Geometry check sheet. Reference: the model listing, model coordinates, mm. Face numbers are marked on the shaded views. A direction names the side the tool comes from. Round coordinates to 2 decimals unless told otherwise and drop trailing zeros. Order: outer loops, then holes, each group sorted by start corner. A loop starts at its lowest first (then second) coordinate and runs counter-clockwise, first axis right, second up. Notation, with made-up numbers: (87.25, -20) - (105.25, -20) arc R19 cw to (105.25, -1) - close; hole circle Ø4 at (16.25, -38). An arc over 180 degrees is marked (long way). Return JSON: item names as keys, results as strings. Group by question number.
Q1. Sectioned sample at B-B, the plane y = 24. Record the cut outline in (x, z).
Q2. Draft check along X on the marked faces 5, 6 and 7. Enter one of: pulls with the +X half, pulls with the -X half, needs draft (parallel to the pull), parting line crosses it, or undercut.
Q3. Sectioned sample at A-A, the plane z = 0. Record the cut outline in (x, y), then the cut area to 3 significant figures.
Q4. Gauge pin test, flat ends, axial feed: pin 1 Ø9.5 at (y, z) = (30, 19) entering from +X; pin 2 Ø10 at (x, z) = (39.5, -13.5) entering from +Y. Record the tip position at first contact, or that the pin passes through.
Q5. Sectioned sample at D-D, the plane y = 5. Record the cut outline in (x, z).
Q6. Material ranges on line 1 along Y through (x, z) = (-35, -15); line 2 along Z through (x, y) = (-18, 50); line 3 along Y through (x, z) = (12, -10.5), recorded low to high.
Q7. Sectioned sample at C-C, the plane x = -35. Record the cut outline in (y, z).
Q8. Tool access check on the marked faces 1, 2, 3 and 4. Record the directions out of +Z, -Z, +X, -X, +Y, -Y that give a thin tool (end or side, any length) a straight path to the whole face; none if there is none.
```python
from build123d import *

# Parameters (mm, degrees)
SKETCH3_R           = 22
BOSS_EXTRUDE1_DEPTH = 16
CUT_EXTRUDE1_DEPTH  = 16
BOSS_EXTRUDE2_DEPTH = 12
FILLET1_R           = 2


with BuildPart() as part:
    # Sketch3 → Boss-Extrude1 (new body)
    with BuildSketch(Plane(origin=(0, 0, 0), x_dir=(1, 0, 0), z_dir=(0, 1, 0))):
        with BuildLine():
            Line((-59, -22), (37, -22))
            ThreePointArc((37, -22), (15, 0), (37, 22))
            Line((37, 22), (-59, 22))
            Line((-59, 22), (-59, -22))
        make_face()
        with Locations((37, 0)):
            Circle(SKETCH3_R)
    extrude(amount=BOSS_EXTRUDE1_DEPTH)

    # Sketch4 → Cut-Extrude1 (cut)
    with BuildSketch(Plane(origin=(0, 16, 0), x_dir=(1, 0, 0), z_dir=(0, 1, 0))):
        with BuildLine():
            Line((37, -8), (13, -8))
            ThreePointArc((13, -8), (5, 0), (13, 8))
            Line((13, 8), (37, 8))
            ThreePointArc((37, 8), (45, 0), (37, -8))
        make_face()
    extrude(amount=-CUT_EXTRUDE1_DEPTH, mode=Mode.SUBTRACT)

    # Sketch5 → Boss-Extrude2 (add)
    with BuildSketch(Plane.XY.offset(22)):
        with BuildLine():
            Line((-59, 40), (-59, 16))
            Line((-59, 16), (-11, 16))
            Line((-11, 16), (-11, 40))
            Line((-11, 40), (-11.018613653, 40))
            ThreePointArc((-11.018613653, 40), (-35, 16.018613653), (-58.981386347, 40))
            Line((-58.981386347, 40), (-59, 40))
        make_face()
        with BuildLine():
            ThreePointArc((-11.018613653, 40), (-35, 63.981386347), (-58.981386347, 40))
            Line((-58.981386347, 40), (-45, 40))
            ThreePointArc((-45, 40), (-35, 50), (-25, 40))
            Line((-25, 40), (-11.018613653, 40))
        make_face()
        with BuildLine():
            Line((-45, 40), (-58.981386347, 40))
            ThreePointArc((-58.981386347, 40), (-35, 16.018613653), (-11.018613653, 40))
            Line((-11.018613653, 40), (-25, 40))
            ThreePointArc((-25, 40), (-35, 30), (-45, 40))
        make_face()
    boss_extrude2 = extrude(amount=-BOSS_EXTRUDE2_DEPTH)

    # Mirror1: Boss-Extrude2 across plane
    add(boss_extrude2.mirror(Plane.XY))

    # Fillet1
    fillet1_edges = [part.edges().sort_by_distance(p)[0] for p in [
        (-11, 16, 16),
        (-35, 16, 10),
        (-35, 16, -10),
        (-11, 16, -16),
    ]]
    fillet(fillet1_edges, radius=FILLET1_R)


solid = part.part
```
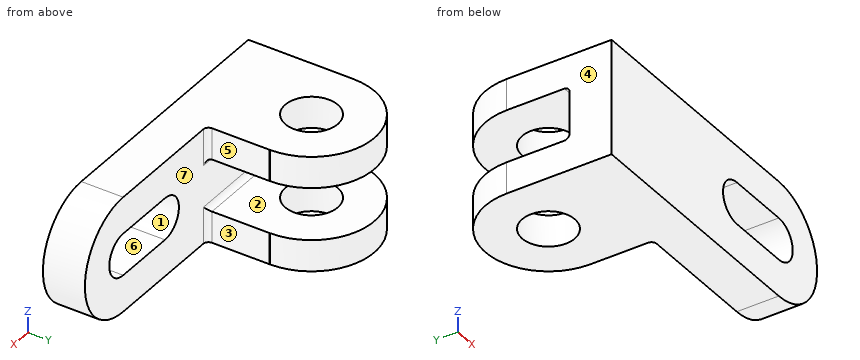
Reply:
{
 "1": {"outline": "(-59, -22) - (-11, -22) - (-11, -10) - (-59, -10) - close; (-59, 10) - (-11, 10) - (-11, 22) - (-59, 22) - close"},
 "2": {"face 5": "pulls with the +X half", "face 6": "undercut", "face 7": "needs draft"},
 "3": {"outline": "(-59, 0) - (5, 0) - (5, 16) - (-59, 16) - close; (45, 0) - (59, 0) - (59, 16) - (45, 16) - close", "area": "1,250 mm^2"},
 "4": {"pin 1": "x = -11", "pin 2": "y = 16"},
 "5": {"outline": "(-59, -22) - (37, -22) arc R22 ccw to (37, 22) - (-59, 22) - close; hole (13, -8) - (37, -8) arc R8 ccw to (37, 8) - (13, 8) arc R8 ccw to start"},
 "6": {"line 1": "0 to 30, 50 to 63.98", "line 2": "-22 to -10, 10 to 22", "line 3": "0 to 16"},
 "7": {"outline": "(0, -22) - (30, -22) - (30, -10) - (18, -10) arc R2 cw to (16, -8) - (16, 8) arc R2 cw to (18, 10) - (30, 10) - (30, 22) - (0, 22) - close; (50, -22) - (63.98, -22) - (63.98, -10) - (50, -10) - close; (50, 10) - (63.98, 10) - (63.98, 22) - (50, 22) - close"},
 "8": {"face 1": "+Y, -Y", "face 2": "+X, -X, +Y", "face 3": "+Z, -Z, +X, +Y", "face 4": "+Z, -Z, -X, +Y, -Y"}
}
